from build123d import *

# Parameters (mm, degrees)
F0_R     = 10.5
F1_DEPTH = 34
F2_DEPTH = 55


with BuildPart() as f1:
    # F0 (on Front) → F1 (new body)
    with BuildSketch(Plane.XZ):
        with BuildLine():
            ThreePointArc((106, 0), (102.753141, 9.992553), (94.252809, 16.168117))
            ThreePointArc((94.252809, 16.168117), (72, 0), (94.252809, -16.168117))
            ThreePointArc((94.252809, -16.168117), (102.753141, -9.992553), (106, 0))
        make_face()
        with Locations((89, 0)):
            Circle(F0_R, mode=Mode.SUBTRACT)
        with BuildLine():
            ThreePointArc((13.75, 42.322423), (36.000868, 26.156978), (44.5, 0))
            ThreePointArc((44.5, 0), (36.000868, -26.156978), (13.75, -42.322423))
            Line((13.75, -42.322423), (94.252809, -16.168117))
            ThreePointArc((94.252809, -16.168117), (72, 0), (94.252809, 16.168117))
            Line((94.252809, 16.168117), (13.75, 42.322423))
        make_face()
        with BuildLine():
            ThreePointArc((13.75, -42.322423), (36.000868, -26.156978), (44.5, 0))
            ThreePointArc((44.5, 0), (36.000868, 26.156978), (13.75, 42.322423))
            ThreePointArc((13.75, 42.322423), (-44.5, 0), (13.75, -42.322423))
        make_face()
        with BuildLine():
            ThreePointArc((-8.246211, 6.5), (0, 10.5), (8.246211, 6.5))
            Line((8.246211, 6.5), (17, 6.5))
            Line((17, 6.5), (17, -6.5))
            Line((17, -6.5), (8.246211, -6.5))
            ThreePointArc((8.246211, -6.5), (0, -10.5), (-8.246211, -6.5))
            Line((-8.246211, -6.5), (-17, -6.5))
            Line((-17, -6.5), (-17, 6.5))
            Line((-17, 6.5), (-8.246211, 6.5))
        make_face(mode=Mode.SUBTRACT)
        with BuildLine():
            ThreePointArc((-8.246211, -6.5), (-10.5, 0), (-8.246211, 6.5))
            Line((-8.246211, 6.5), (-17, 6.5))
            Line((-17, 6.5), (-17, -6.5))
            Line((-17, -6.5), (-8.246211, -6.5))
        make_face()
    extrude(amount=F1_DEPTH)

    # F0 (on Front) → F2 (join)
    with BuildSketch(Plane.XZ):
        with BuildLine():
            ThreePointArc((13.75, -42.322423), (36.000868, -26.156978), (44.5, 0))
            ThreePointArc((44.5, 0), (36.000868, 26.156978), (13.75, 42.322423))
            ThreePointArc((13.75, 42.322423), (-44.5, 0), (13.75, -42.322423))
        make_face()
        with BuildLine():
            ThreePointArc((-8.246211, 6.5), (0, 10.5), (8.246211, 6.5))
            Line((8.246211, 6.5), (17, 6.5))
            Line((17, 6.5), (17, -6.5))
            Line((17, -6.5), (8.246211, -6.5))
            ThreePointArc((8.246211, -6.5), (0, -10.5), (-8.246211, -6.5))
            Line((-8.246211, -6.5), (-17, -6.5))
            Line((-17, -6.5), (-17, 6.5))
            Line((-17, 6.5), (-8.246211, 6.5))
        make_face(mode=Mode.SUBTRACT)
        with BuildLine():
            ThreePointArc((-8.246211, -6.5), (-10.5, 0), (-8.246211, 6.5))
            Line((-8.246211, 6.5), (-17, 6.5))
            Line((-17, 6.5), (-17, -6.5))
            Line((-17, -6.5), (-8.246211, -6.5))
        make_face()
    extrude(amount=F2_DEPTH)


solid = f1.part
Can you work these out from the model? Positions are in its coordinate system, mm. A direction names the side the tool comes from. Give positions to 0.01 mm unless a question says otherwise; leave off trailing zeros. Write each loop counter-clockwise with the first axis right and the second up, starting at its lowest first coordinate (ties: lowest second). Pieces come first, ordered by that corner, then holes. Notation, with made-up numbers: M 46,5 L 74,5 A17 cw 74,35 Z; hole C -15,17 d4. An arc over 180 degrees is marked long. Answer in a Markdown table with one row per item. Add a question column.
Item 1: Please list where these lines run through material, in increasing order: L1, parallel to X at y = -16.5, z = 0.5; L2, parallel to Z at x = 0, y = -36.5; L3, parallel to Z at x = 89, y = -10.
Item 2: Imagine slicing it at A-A, the plane y = -30.5. Write out the boundary of the cut face in (x, z).
Item 3: On a 3-axis mill with a long thin cutter (end or side, diameter ignored), from which of +Z, -Z, +X, -X, +Y, -Y can I reach the whole of each face in a straight line? I mean faces 5 (the flat face through (54.565, -16.762, 29.062)), 6 (the flat face through (13, -27, -6.5)). Say none if no direction works.
Item 4: Imagine slicing it at B-B, the plane x = 0. Write out the boundary of the cut face in (y, z).
Item 5: For pin 1 Ø8 at (x, z) = (58, -24.5) entering from -Y; pin 2 Ø7 at (x, y) = (14, -30.5) entering from +Z; pin 3 Ø8 at (x, y) = (-21, -12.5) entering from +Z; pin 4 Ø10 at (y, z) = (-11.5, 3) entering from -X, each with a flat end and sliding along its axis, tell me the tip position at first contact or that it passes through.
Item 6: We'd pull the mould along X, two halves only. Please class faces 1 (the flat face through (17, -27, 0)), 2 (the flat face through (13, -27, 6.5)), 3 (the flat face through (63, -34, 3)), 4 (the flat face through (53.438, -16.762, -29.428)): released by +X, released by -X, zero draft, split by the parting line, or undercut.
Item 7: Imagine slicing it at D-D, the plane x = 91.5. Write out the boundary of the cut face in (y, z), plus the area to 3 significant figures.
Item 8: Imagine slicing it at C-C, the plane y = -48. Write out the boundary of the cut face in (x, z).
Evaluation:
| question | item | result |
|---|---|---|
| 1 | L1 | x = -44.5 to -10.49, 17 to 78.51, 99.49 to 105.99 |
| 1 | L2 | z = -44.5 to -10.5, 10.5 to 44.5 |
| 1 | L3 | z = -17.87 to -10.5, 10.5 to 17.87 |
| 2 | outline | M 13.75,-42.32 L 94.25,-16.17 A17 ccw 94.25,16.17 L 13.75,42.32 A44.5 ccw long Z; hole M 8.25,-6.5 L 17,-6.5 L 17,6.5 L 8.25,6.5 A10.5 ccw long Z; hole C 89,0 d21 |
| 3 | face 5 | +Z, +X, +Y, -Y |
| 3 | face 6 | +Y, -Y |
| 4 | outline | M -55,-44.5 L 0,-44.5 L 0,-10.5 L -55,-10.5 Z; M -55,10.5 L 0,10.5 L 0,44.5 L -55,44.5 Z |
| 5 | pin 1 | stops at y = -34 |
| 5 | pin 2 | stops at z = 43.24 |
| 5 | pin 3 | stops at z = 41.12 |
| 5 | pin 4 | stops at x = -44.5 |
| 6 | face 1 | undercut |
| 6 | face 2 | undercut |
| 6 | face 3 | zero draft |
| 6 | face 4 | released by +X |
| 7 | outline | M -34,-17.06 L 0,-17.06 L 0,-10.2 L -34,-10.2 Z; M -34,10.2 L 0,10.2 L 0,17.06 L -34,17.06 Z |
| 7 | area | 467 mm² |
| 8 | outline | C 0,0 d89; hole M 8.25,-6.5 L 17,-6.5 L 17,6.5 L 8.25,6.5 A10.5 ccw long Z |
